Could you check a few things on this model? Use its own coordinates, in mm. A direction names the side the tool comes from. Coordinates: 2 decimals unless noted, no trailing zeros. Order: outer loops, then holes, each group sorted by start corner. A loop starts at its lowest first (then second) coordinate and runs counter-clockwise, first axis right, second up. Notation, with made-up numbers: (-9, -35.75) -> (45, -35.75) arc R19 cw to (45, -25.75) -> close; hole circle Ø5 at (9, 77.25). An arc over 180 degrees is marked (long way). Use a Markdown table: item, result. Add a question column.
1) If I drill on L1, parallel to Y at x = -6, z = 40; L2, parallel to X at y = -2.7, z = 47.5; L3, parallel to Z at x = -1.5, y = -3.75, over which ranges is the centre line in solid material (lowest first)? Write a range as [from, to].
2) Which directions (+Z, -Z, +X, -X, +Y, -Y) give clear straight access to the entire face, cutting with the end or side of a thin tool? Please do faces 5 (the flat face through (0, 3, 15)), 6 (the flat face through (0, -6, 38)), 7 (the flat face through (0, 4.3, 44)).
3) Will these pins go through, and if not, where does the flat tip stop? pin 1 Ø7.5 at (x, z) = (0.5, 48) entering from -Y; pin 2 Ø5.5 at (x, z) = (0, 7.5) entering from +Y; pin 3 Ø5 at (x, y) = (0, -1) entering from +Z; pin 4 Ø1.6 at (x, y) = (-0.5, 6.5) entering from +Z.
4) If we section it at C-C (y = -2.25): Write out the boundary of the cut face in (x, z), plus the area to 3 significant figures.
5) Thinking about a two-plate mould opening in Y: for faces 1 (the flat face through (0, -4.3, 44)), 2 (the flat face through (7.5, -2, 23)), 3 (the flat face through (0, 1.7, 44)), 4 (the flat face through (0, -1.7, 44)), which applies, +Y half, -Y half, draft (parallel to the pull), parting line (faces both ways), or undercut?
6) If we section it at D-D (y = 2.75): Write out the boundary of the cut face in (x, z).
7) If we section it at A-A (z = 7.5): Write out the boundary of the cut face in (x, y), plus the area to 3 significant figures.
8) If we section it at B-B (x = 0): Write out the boundary of the cut face in (y, z).
```python
from build123d import *

# Parameters (mm, degrees)
CYLINDER005_R     = 2.2
CYLINDER005_DEPTH = 6
BOX008_W          = 15
BOX008_H          = 6
BOX008_DEPTH      = 15
CYLINDER004_R     = 1.9
CYLINDER004_DEPTH = 15
BOX005_W          = 15
BOX005_H          = 3.4
BOX005_DEPTH      = 17
ARRAY001_Y_COUNT  = 3
ARRAY001_Y_PITCH  = 6
CYLINDER003_R     = 7.5
CYLINDER003_DEPTH = 15
BOX004_W          = 15
BOX004_H          = 15
BOX004_DEPTH      = 12.5
BOX009_W          = 15
BOX009_H          = 15
BOX009_DEPTH      = 20


with BuildPart() as insert_hole001:
    # Cylinder005 → Cylinder005 (new body)
    with BuildSketch(Plane(origin=(0, -1.5, 7.5), x_dir=(1, 0, 0), z_dir=(0, -1, 0))):
        Circle(CYLINDER005_R)
    extrude(amount=CYLINDER005_DEPTH)


with BuildPart() as one_cube_with_insert_hole_cut:
    # Box008 → Box008 (new body)
    with BuildSketch(Plane(origin=(-7.5, -7.5, 0), x_dir=(1, 0, 0), z_dir=(0, 0, 1))):
        with Locations((7.5, 3)):
            Rectangle(BOX008_W, BOX008_H)
    extrude(amount=BOX008_DEPTH)

    # Cut004: cut insert hole001
    add(insert_hole001.part, mode=Mode.SUBTRACT)


with BuildPart() as side_2_bolt_hole:
    # Cylinder004 → Cylinder004 (new body)
    with BuildSketch(Plane(origin=(0, 7.5, 12.5), x_dir=(1, 0, 0), z_dir=(0, -1, 0))):
        Circle(CYLINDER004_R)
    extrude(amount=CYLINDER004_DEPTH)


with BuildPart() as side_2_extract_fusion:
    # Box005 → Box005 (new body)
    with BuildSketch(Plane(origin=(-7.5, -7.7, 3), x_dir=(1, 0, 0), z_dir=(0, 0, 1))):
        with Locations((7.5, 1.7)):
            Rectangle(BOX005_W, BOX005_H)
    extrude(amount=BOX005_DEPTH)

    # Array001 Y: side 2 extract fusion ×3


with BuildPart() as side_2_extract_fusion_1:
    add(side_2_extract_fusion.part)
    with Locations(*[(0, i * ARRAY001_Y_PITCH, 0) for i in range(1, ARRAY001_Y_COUNT)]):
        add(side_2_extract_fusion.part)

    # Fusion004: union side 2 bolt hole
    add(side_2_bolt_hole.part)


with BuildPart() as outer_cylinder001:
    # Cylinder003 → Cylinder003 (new body)
    with BuildSketch(Plane(origin=(0, 7.5, 12.5), x_dir=(1, 0, 0), z_dir=(0, -1, 0))):
        Circle(CYLINDER003_R)
    extrude(amount=CYLINDER003_DEPTH)


with BuildPart() as side_2_cut_clone001:
    # Box004 → Box004 (new body)
    with BuildSketch(Plane(origin=(-7.5, -7.5, 0), x_dir=(1, 0, 0), z_dir=(0, 0, 1))):
        with Locations((7.5, 7.5)):
            Rectangle(BOX004_W, BOX004_H)
    extrude(amount=BOX004_DEPTH)

    # Fusion003: union outer cylinder001
    add(outer_cylinder001.part)

    # Cut001: cut side 2 extract fusion
    add(side_2_extract_fusion_1.part, mode=Mode.SUBTRACT)


with BuildPart() as side_2_cut_clone001_1:
    # Body004 placement: moved
    add(side_2_cut_clone001.part.moved(Location((0, 0, 35))))


with BuildPart() as side_2_one_fusion00:
    # Box009 → Box009 (new body)
    with BuildSketch(Plane(origin=(-7.5, -7.5, 15), x_dir=(1, 0, 0), z_dir=(0, 0, 1))):
        with Locations((7.5, 7.5)):
            Rectangle(BOX009_W, BOX009_H)
    extrude(amount=BOX009_DEPTH)

    # Fusion006: union one cube with insert hole cut, side 2 cut clone001
    add(one_cube_with_insert_hole_cut.part)
    add(side_2_cut_clone001_1.part)


solid = side_2_one_fusion00.part
```
Answer sheet:
| question | item | result |
|---|---|---|
| 1 | L1 | [-4.3, -1.7], [1.7, 4.3] |
| 1 | L2 | [-7.5, -1.9], [1.9, 7.5] |
| 1 | L3 | [0, 5.89], [9.11, 46.33], [48.67, 54.85] |
| 2 | face 5 | -Z, +X, -X, +Y |
| 2 | face 6 | +Z, +X, -X, -Y |
| 2 | face 7 | +Z, +X, -X, +Y |
| 3 | pin 1 | y = -4.3 |
| 3 | pin 2 | y = -1.5 |
| 3 | pin 3 | z = 55 |
| 3 | pin 4 | z = 38 |
| 4 | outline | (-7.5, 0) -> (7.5, 0) -> (7.5, 47.5) arc R7.5 ccw to (-7.5, 47.5) -> close; hole circle Ø4.4 at (0, 7.5); hole circle Ø3.8 at (0, 47.5) |
| 4 | area | 774 mm2 |
| 5 | face 1 | -Y half |
| 5 | face 2 | draft |
| 5 | face 3 | undercut |
| 5 | face 4 | undercut |
| 6 | outline | (-7.5, 15) -> (7.5, 15) -> (7.5, 47.5) arc R7.5 ccw to (-7.5, 47.5) -> close; hole circle Ø3.8 at (0, 47.5) |
| 7 | outline | (-7.5, -7.5) -> (-2.2, -7.5) -> (-2.2, -1.5) -> (-7.5, -1.5) -> close; (2.2, -7.5) -> (7.5, -7.5) -> (7.5, -1.5) -> (2.2, -1.5) -> close |
| 7 | area | 63.6 mm2 |
| 8 | outline | (-7.5, 0) -> (-1.5, 0) -> (-1.5, 5.3) -> (-7.5, 5.3) -> close; (-7.5, 9.7) -> (-1.5, 9.7) -> (-1.5, 15) -> (7.5, 15) -> (7.5, 38) -> (4.3, 38) -> (4.3, 45.6) -> (1.7, 45.6) -> (1.7, 38) -> (-1.7, 38) -> (-1.7, 45.6) -> (-4.3, 45.6) -> (-4.3, 38) -> (-7.5, 38) -> close; (-4.3, 49.4) -> (-1.7, 49.4) -> (-1.7, 55) -> (-4.3, 55) -> close; (1.7, 49.4) -> (4.3, 49.4) -> (4.3, 55) -> (1.7, 55) -> close |
